Geometry: final body of the model. Coordinates: model frame, mm. Face numbers are marked on the shaded views. A direction names the side the tool comes from. Coordinates: 2 decimals unless noted, no trailing zeros. Write each loop counter-clockwise with the first axis right and the second up, starting at its lowest first coordinate (ties: lowest second). Pieces come first, ordered by that corner, then holes. Notation, with made-up numbers: (52.5, 17.5) -> (111.5, 17.5) arc R28 ccw to (111.5, 45.5) -> close; hole circle Ø9 at (-18, -36). An arc over 180 degrees is marked (long way). One line per item, written item: value.
```python
from build123d import *

# Parameters (mm, degrees)
PAD023_DEPTH    = 144
SKETCH036_R     = 1.5
POCKET004_DEPTH = 4
SKETCH037_R     = 2.75
POCKET005_DEPTH = 2


with BuildPart() as left:
    # Sketch035 → Pad023 (new body)
    with BuildSketch(Plane.XZ):
        Polygon((0, 0), (0, -4), (10, -4), (10, -31), (0, -31), (0, -35), (32, -35), (32, -31), (14, -31), (14, -4), (14, 0), align=None)
    extrude(amount=PAD023_DEPTH)

    # Sketch036 (on Face12 of Pad023) → Pocket004 (cut)
    with BuildSketch(Plane(origin=(14, 0, 0), x_dir=(0, 0, 1), z_dir=(1, 0, 0))):
        with Locations((-7.5, 118.15)):
            Circle(SKETCH036_R)
        with Locations((-7.5, 103.15)):
            Circle(SKETCH036_R)
        with Locations((-27.5, 103.15)):
            Circle(SKETCH036_R)
        with Locations((-27.5, 118.15)):
            Circle(SKETCH036_R)
        with Locations((-27.5, 40.85)):
            Circle(SKETCH036_R)
        with Locations((-27.5, 25.85)):
            Circle(SKETCH036_R)
        with Locations((-7.5, 25.85)):
            Circle(SKETCH036_R)
        with Locations((-7.5, 40.85)):
            Circle(SKETCH036_R)
    extrude(amount=-POCKET004_DEPTH, mode=Mode.SUBTRACT)

    # Sketch037 (on Face6 of Pocket004) → Pocket005 (cut)
    with BuildSketch(Plane(origin=(14, 0, 0), x_dir=(0, 0, 1), z_dir=(1, 0, 0))):
        with Locations((-7.5, 118.15)):
            Circle(SKETCH037_R)
        with Locations((-7.5, 103.15)):
            Circle(SKETCH037_R)
        with Locations((-27.5, 103.15)):
            Circle(SKETCH037_R)
        with Locations((-27.5, 118.15)):
            Circle(SKETCH037_R)
        with Locations((-27.5, 40.85)):
            Circle(SKETCH037_R)
        with Locations((-27.5, 25.85)):
            Circle(SKETCH037_R)
        with Locations((-7.5, 25.85)):
            Circle(SKETCH037_R)
        with Locations((-7.5, 40.85)):
            Circle(SKETCH037_R)
    extrude(amount=-POCKET005_DEPTH, mode=Mode.SUBTRACT)


with BuildPart() as left_1:
    # Body011 placement: moved
    add(left.part.moved(Location((-66, -59.5, 31))))


with BuildPart() as right:
    # Part__Mirroring: instance of Left
    add(left_1.part.mirror(Plane(origin=(0, 0, 0), x_dir=(0, -1, 0), z_dir=(1, 0, 0))))


solid = right.part
```
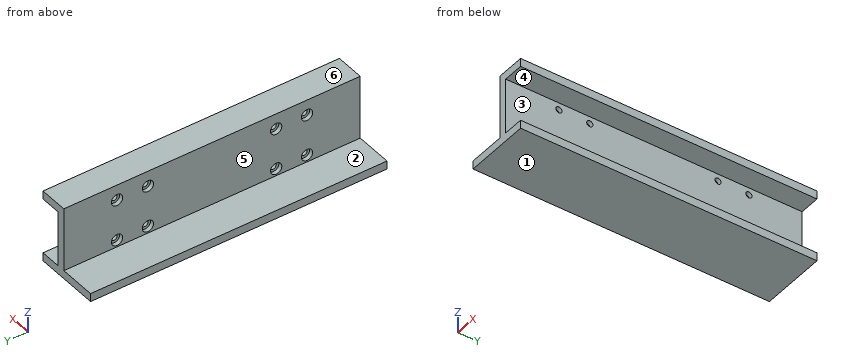
(1) Reachability of the marked faces 4, 5 and 6 from +Z, -Z, +X, -X, +Y, -Y: full face, straight path, thin tool, end or side. Return the list, or none.
Responses:
face 4: +X, +Y, -Y
face 5: +Z, -X, +Y, -Y
face 6: +Z, +X, -X, +Y, -Y
(2) Section D-D (z = 23.5). State how many separate pieces and enclosed holes the cut face has, then the cut area to 3 significant figures.
Responses:
separate pieces: 5
enclosed holes: 0
area: 508 mm2
(3) Section C-C (y = -139.5). Return the cut outline in (x, z), then the cut area to 3 significant figures.
Responses:
outline: (34, -4) -> (66, -4) -> (66, 0) -> (56, 0) -> (56, 27) -> (66, 27) -> (66, 31) -> (52, 31) -> (52, 0) -> (34, 0) -> close
area: 292 mm2
(4) Section A-A (y = -85.35). Return the cut outline in (x, z).
Responses:
outline: (34, -4) -> (66, -4) -> (66, 0) -> (56, 0) -> (56, 2) -> (54, 2) -> (54, 0.75) -> (52, 0.75) -> (52, 0) -> (34, 0) -> close; (52, 6.25) -> (54, 6.25) -> (54, 5) -> (56, 5) -> (56, 22) -> (54, 22) -> (54, 20.75) -> (52, 20.75) -> close; (52, 26.25) -> (54, 26.25) -> (54, 25) -> (56, 25) -> (56, 27) -> (66, 27) -> (66, 31) -> (52, 31) -> close
(5) Pull-direction query (Z, two-part tool) for the marked faces 1, 2 and 3; classes: released by +Z, released by -Z, zero draft, split by the parting line, or undercut.
Responses:
face 1: released by -Z
face 2: released by +Z
face 3: undercut
(6) First-contact query: pin 1 (3.5 mm diameter, centred on y = -85.35, z = 23.5, fed in from -X); pin 2 (3.5 mm diameter, centred on y = -100.35, z = 3.5, fed in from +X); pin 3 (1.5 mm diameter, centred on y = -178, z = 9.5, fed in from -X); pin 4 (2.5 mm diameter, centred on y = -162.65, z = 23.5, fed in from +X). Flat tips, straight axial feed; report the tip coordinate or a pass-through.
Responses:
pin 1: stops at x = 54
pin 2: stops at x = 56
pin 3: stops at x = 52
pin 4: passes through
(7) Section B-B (x = 59.5). Return the cut outline in (y, z), then the cut area to 3 significant figures.
Responses:
outline: (-203.5, -4) -> (-59.5, -4) -> (-59.5, 0) -> (-203.5, 0) -> close; (-203.5, 27) -> (-59.5, 27) -> (-59.5, 31) -> (-203.5, 31) -> close
area: 1,150 mm2
(8) Line query: line 1 (Z direction, x = 53.45, y = -100.35); line 2 (Z direction, x = 55.3, y = -162.65); line 3 (Y direction, x = 55.4, z = 3.5). Output: solid intervals per line, ascending. Write a range as [from, to].
Responses:
line 1: z = [-4, 0.75], [6.25, 20.75], [26.25, 31]
line 2: z = [-4, 2], [5, 22], [25, 31]
line 3: y = [-203.5, -179.15], [-176.15, -164.15], [-161.15, -101.85], [-98.85, -86.85], [-83.85, -59.5]
